For this review, take the finished solid that the model builds, in its own axes (mm). Give positions to 0.01 mm unless a question says otherwise; leave off trailing zeros. Order: outer loops, then holes, each group sorted by start corner. A loop starts at its lowest first (then second) coordinate and runs counter-clockwise, first axis right, second up. Notation, with made-up numbers: (0.25, 45.5) - (22.25, 45.5) arc R14 cw to (22.25, 70.5) - close; hole circle Ø9 at (32.25, -37.75). An arc over 180 degrees is marked (long way). Put each result on its own line as item: value. Start each with the question number.
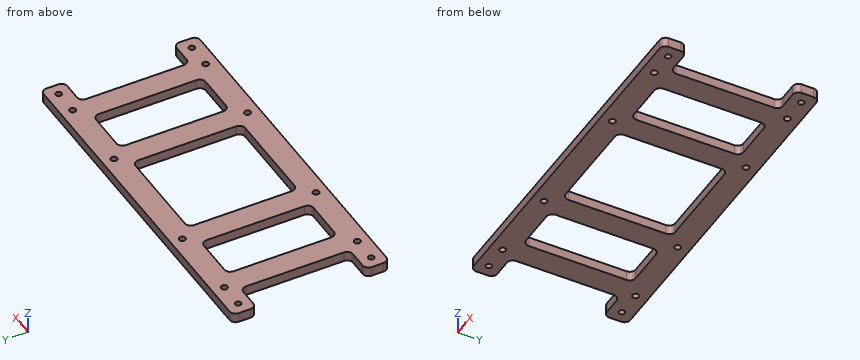
```python
from build123d import *

# Parameters (mm, degrees)
EXTRUDE_1_DEPTH     = 5
FILLET_1_R          = 3
SKETCH_2_R          = 1.5
SKETCH_2_R_2        = 1.6
CUT_EXTRUDE_1_DEPTH = 7
SKETCH_3_W          = 12
SKETCH_3_H          = 55.843243592
EXTRUDE_2_DEPTH     = 5
FILLET_2_R          = 3


with BuildPart() as part:
    # 草图1 → 凸台-拉伸1 (new body)
    with BuildSketch(Plane.XY):
        with BuildLine():
            Line((-20, 39.843243592), (154, 39.843243592))
            ThreePointArc((154, 39.843243592), (156.121320344, 38.964563935), (157, 36.843243592))
            Line((157, 36.843243592), (157, 30.843243592))
            ThreePointArc((157, 30.843243592), (156.121320344, 28.721923248), (154, 27.843243592))
            Line((154, 27.843243592), (142, 27.843243592))
            Line((142, 27.843243592), (142, -28))
            Line((142, -28), (154, -28))
            ThreePointArc((154, -28), (156.121320344, -28.878679656), (157, -31))
            Line((157, -31), (157, -37))
            ThreePointArc((157, -37), (156.121320344, -39.121320344), (154, -40))
            Line((154, -40), (-20, -40))
            ThreePointArc((-20, -40), (-22.121320344, -39.121320344), (-23, -37))
            Line((-23, -37), (-23, -31))
            ThreePointArc((-23, -31), (-22.121320344, -28.878679656), (-20, -28))
            Line((-20, -28), (-8, -28))
            Line((-8, -28), (-8, 27.843243592))
            Line((-8, 27.843243592), (-20, 27.843243592))
            ThreePointArc((-20, 27.843243592), (-22.121320344, 28.721923248), (-23, 30.843243592))
            Line((-23, 30.843243592), (-23, 36.843243592))
            ThreePointArc((-23, 36.843243592), (-22.121320344, 38.964563935), (-20, 39.843243592))
        make_face()
        with BuildLine():
            ThreePointArc((7, 27.843243592), (4.878679656, 26.964563935), (4, 24.843243592))
            Line((4, 24.843243592), (4, -25))
            ThreePointArc((4, -25), (4.878679656, -27.121320344), (7, -28))
            Line((7, -28), (127, -28))
            ThreePointArc((127, -28), (129.121320344, -27.121320344), (130, -25))
            Line((130, -25), (130, 24.843243592))
            ThreePointArc((130, 24.843243592), (129.121320344, 26.964563935), (127, 27.843243592))
            Line((127, 27.843243592), (7, 27.843243592))
        make_face(mode=Mode.SUBTRACT)
    extrude(amount=EXTRUDE_1_DEPTH)

    # 圆角1
    fillet_1_edges = [part.edges().sort_by_distance(p)[0] for p in [
        (142, 27.843243592, 2.5),
        (142, -28, 2.5),
        (-8, -28, 2.5),
        (-8, 27.843243592, 2.5),
    ]]
    fillet(fillet_1_edges, radius=FILLET_1_R)

    # 草图2 → 切除-拉伸1 (cut)
    with BuildSketch(Plane.XY.offset(5)):
        with Locations((-16.977965312, 33.843243592)):
            Circle(SKETCH_2_R)
        with Locations((-4, 33.843243592)):
            Circle(SKETCH_2_R_2)
        with Locations((35.001599808, 34)):
            Circle(SKETCH_2_R_2)
        with Locations((98.998400192, 34)):
            Circle(SKETCH_2_R_2)
        with Locations((138, 33.843243592)):
            Circle(SKETCH_2_R_2)
        with Locations((150.977965312, 33.843243592)):
            Circle(SKETCH_2_R)
        with Locations((150.977965312, -34)):
            Circle(SKETCH_2_R)
        with Locations((138, -34)):
            Circle(SKETCH_2_R_2)
        with Locations((98.998400192, -34.156756408)):
            Circle(SKETCH_2_R_2)
        with Locations((35.001599808, -34.156756408)):
            Circle(SKETCH_2_R_2)
        with Locations((-4, -34)):
            Circle(SKETCH_2_R_2)
        with Locations((-16.977965312, -34)):
            Circle(SKETCH_2_R)
    extrude(amount=-CUT_EXTRUDE_1_DEPTH, mode=Mode.SUBTRACT)

    # 草图3 → 凸台-拉伸2 (add)
    with BuildSketch(Plane(origin=(0, 0, 0), x_dir=(-1, 0, 0), z_dir=(0, 0, -1))):
        with Locations((-98.998400192, -0.078378204)):
            Rectangle(SKETCH_3_W, SKETCH_3_H)
        with Locations((-35.001599808, -0.078378204)):
            Rectangle(SKETCH_3_W, SKETCH_3_H)
    extrude(amount=-EXTRUDE_2_DEPTH)

    # 圆角2
    fillet_2_edges = [part.edges().sort_by_distance(p)[0] for p in [
        (104.998400192, -28, 2.5),
        (104.998400192, 27.843243592, 2.5),
        (92.998400192, 27.843243592, 2.5),
        (92.998400192, -28, 2.5),
        (41.001599808, -28, 2.5),
        (41.001599808, 27.843243592, 2.5),
        (29.001599808, 27.843243592, 2.5),
        (29.001599808, -28, 2.5),
    ]]
    fillet(fillet_2_edges, radius=FILLET_2_R)


solid = part.part
```
1. Wall thickness on line 1 (X direction, y = -14, z = 0.9); line 2 (Y direction, x = 138, z = 2.1); line 3 (Y direction, x = 80, z = 3.4): over which ranges is each line inside the solid? List them lowest first. Write a range as from..to.
2. Add section B-B, the plane x = 59.5. Give the boundary of the cut face in (y, z).
3. Clearance check with flat-ended pins moving along their axes: pin 1 (5 mm diameter, centred on x = 35, y = 34, fed in from +Z); pin 2 (3 mm diameter, centred on y = 5.5, z = 3.5, fed in from -X); pin 3 (2.5 mm diameter, centred on y = 8.5, z = 2, fed in from +X). State where each tip first meets the part, or that it passes through.
4. Add section C-C, the plane x = 138. Give the boundary of the cut face in (y, z), then the cut area to 3 significant figures.
5. Add section D-D, the plane z = 2.85. Count the separate pieces of the cut face and the enclosed holes in it, then the cut area to 3 significant figures.
6. Add section A-A, the plane y = 2.5. Give the boundary of the cut face in (x, z), then the cut area to 3 significant figures.
Found:
1. line 1: x = -8..4, 29..41, 93..105, 130..142
1. line 2: y = -40..-35.6, -32.4..32.24, 35.44..39.84
1. line 3: y = -40..-28, 27.84..39.84
2. outline: (-40, 0) - (-28, 0) - (-28, 5) - (-40, 5) - close; (27.84, 0) - (39.84, 0) - (39.84, 5) - (27.84, 5) - close
3. pin 1: stops at z = 5
3. pin 2: stops at x = -8
3. pin 3: stops at x = 142
4. outline: (-40, 0) - (-35.6, 0) - (-35.6, 5) - (-40, 5) - close; (-32.4, 0) - (32.24, 0) - (32.24, 5) - (-32.4, 5) - close; (35.44, 0) - (39.84, 0) - (39.84, 5) - (35.44, 5) - close
4. area: 367 mm^2
5. separate pieces: 1
5. enclosed holes: 15
5. area: 6,920 mm^2
6. outline: (-8, 0) - (4, 0) - (4, 5) - (-8, 5) - close; (29, 0) - (41, 0) - (41, 5) - (29, 5) - close; (93, 0) - (105, 0) - (105, 5) - (93, 5) - close; (130, 0) - (142, 0) - (142, 5) - (130, 5) - close
6. area: 240 mm^2
